from build123d import *

# Parameters (mm, degrees)
SKETCH1_W                                  = 38
SKETCH1_H                                  = 18
BOSS_EXTRUDE1_DEPTH                        = 34
BOSS_EXTRUDE2_START                        = -6
SKETCH2_W                                  = 54
SKETCH2_H                                  = 18
BOSS_EXTRUDE2_DEPTH                        = 2
CUT_EXTRUDE1_DEPTH                         = 48
CUT_EXTRUDE1_DEPTH_BACK                    = 48
SKETCH3_W                                  = 1.5
SKETCH3_H                                  = 1
SKETCH4_R                                  = 6
BOSS_EXTRUDE3_DEPTH                        = 1.5
SKETCH5_W                                  = 6
SKETCH5_H                                  = 2
BOSS_EXTRUDE4_DEPTH                        = 1
FILLET1_RADIUS                             = 1
FILLET1_LENGTH                             = 1
FILLET1_OF_MIRROR1_2_RADIUS                = 1
FILLET1_OF_MIRROR1_2_LENGTH                = 1
SKETCH6_W                                  = 7
SKETCH6_H                                  = 4
BOSS_EXTRUDE5_DEPTH                        = 5
SKETCH7_R                                  = 3
BOSS_EXTRUDE6_DEPTH                        = 4
BOSS_EXTRUDE7_START                        = 8
SKETCH8_R                                  = 7
BOSS_EXTRUDE7_DEPTH                        = 2
SKETCH9_R                                  = 4
BOSS_EXTRUDE8_DEPTH                        = 4
SKETCH10_R                                 = 2.25
CUT_EXTRUDE2_DEPTH                         = 4
MIRROR2_AT_THE_SECOND_PLANE_COPY_1_SKETC_R = 2.25
MIRROR2_AT_THE_SECOND_PLANE_COPY_1_DEPTH   = 4


with BuildPart() as part:
    # Sketch1 → Boss-Extrude1 (new body)
    with BuildSketch(Plane(origin=(0, 0, 0), x_dir=(1, 0, 0), z_dir=(0, 1, 0))):
        Rectangle(SKETCH1_W, SKETCH1_H)
    extrude(amount=BOSS_EXTRUDE1_DEPTH)

    # Sketch2 → Boss-Extrude2 (add)
    with BuildSketch(Plane(origin=(0, 34, 0), x_dir=(1, 0, 0), z_dir=(0, 1, 0)).offset(BOSS_EXTRUDE2_START)):
        Rectangle(SKETCH2_W, SKETCH2_H)
    extrude(amount=-BOSS_EXTRUDE2_DEPTH)

    # Sketch3 → Cut-Extrude1 (cut, two sides: drawn at the far end of the back side and taken through both)
    with BuildSketch(Plane.XY.offset(9).offset(-CUT_EXTRUDE1_DEPTH_BACK)):
        Polygon((-19, 30), (-16, 31), (-14, 34), (-19, 34), align=None)
        with Locations((-1.75, 33.5)):
            Rectangle(SKETCH3_W, SKETCH3_H)
    extrude(amount=CUT_EXTRUDE1_DEPTH + CUT_EXTRUDE1_DEPTH_BACK, mode=Mode.SUBTRACT)

    # Sketch4 → Boss-Extrude3 (add)
    with BuildSketch(Plane(origin=(0, 34, 0), x_dir=(1, 0, 0), z_dir=(0, 1, 0))):
        with Locations(Location((10, 0, 0), (0, 0, 90))):
            Circle(SKETCH4_R)
    extrude(amount=BOSS_EXTRUDE3_DEPTH)

    # Sketch5 → Boss-Extrude4 (add)
    with BuildSketch(Plane(origin=(0, 28, 0), x_dir=(1, 0, 0), z_dir=(0, 1, 0))):
        with Locations((-22, 0)):
            Rectangle(SKETCH5_W, SKETCH5_H)
    boss_extrude4 = extrude(amount=BOSS_EXTRUDE4_DEPTH)

    # Fillet1: full round fillet: the end face becomes a half cylinder, R = half its width
    fillet1_face = Plane((-25, 28.5, 0), x_dir=(0, -1, 0), z_dir=(-1, 0, 0))  # on the end face: x along it, z out of the body
    fillet1_slab = fillet1_face.offset(-FILLET1_RADIUS / 2) * Box(FILLET1_LENGTH, 2 * FILLET1_RADIUS, FILLET1_RADIUS, mode=Mode.PRIVATE)  # the body's end, R deep
    fillet1_round = Plane((-24, 28.5, 0), x_dir=(-1, 0, 0), z_dir=(0, -1, 0)) * Cylinder(FILLET1_RADIUS, FILLET1_LENGTH, mode=Mode.PRIVATE)  # its axis R under the face
    add(fillet1_slab - fillet1_round, mode=Mode.SUBTRACT)

    # Mirror1: Boss-Extrude4 across plane
    add(boss_extrude4.mirror(Plane(origin=(0, 0, 0), x_dir=(0, 0, 1), z_dir=(1, 0, 0))))

    # Fillet1 of Mirror1 2: full round fillet: the end face becomes a half cylinder, R = half its width
    fillet1_of_mirror1_2_face = Plane((25, 28.5, 0), x_dir=(0, -1, 0), z_dir=(1, 0, 0))  # on the end face: x along it, z out of the body
    fillet1_of_mirror1_2_slab = fillet1_of_mirror1_2_face.offset(-FILLET1_OF_MIRROR1_2_RADIUS / 2) * Box(FILLET1_OF_MIRROR1_2_LENGTH, 2 * FILLET1_OF_MIRROR1_2_RADIUS, FILLET1_OF_MIRROR1_2_RADIUS, mode=Mode.PRIVATE)  # the body's end, R deep
    fillet1_of_mirror1_2_round = Plane((24, 28.5, 0), x_dir=(1, 0, 0), z_dir=(0, -1, 0)) * Cylinder(FILLET1_OF_MIRROR1_2_RADIUS, FILLET1_OF_MIRROR1_2_LENGTH, mode=Mode.PRIVATE)  # its axis R under the face
    add(fillet1_of_mirror1_2_slab - fillet1_of_mirror1_2_round, mode=Mode.SUBTRACT)

    # Sketch6 → Boss-Extrude5 (add)
    with BuildSketch(Plane(origin=(19, 0, 0), x_dir=(0, 0, -1), z_dir=(1, 0, 0))):
        with Locations((0, 3)):
            Rectangle(SKETCH6_W, SKETCH6_H)
    extrude(amount=BOSS_EXTRUDE5_DEPTH)

    # Sketch7 → Boss-Extrude6 (add)
    with BuildSketch(Plane(origin=(0, 35.5, 0), x_dir=(1, 0, 0), z_dir=(0, 1, 0))):
        with Locations(Location((10, 0, 0), (0, 0, 270))):
            Circle(SKETCH7_R)
    extrude(amount=BOSS_EXTRUDE6_DEPTH)



with BuildPart() as body_2:
    # Sketch8 → Boss-Extrude7 (new body)
    with BuildSketch(Plane(origin=(0, 34, 0), x_dir=(1, 0, 0), z_dir=(0, 1, 0)).offset(BOSS_EXTRUDE7_START)):
        with Locations(Location((10, 0, 0), (0, 0, 270))):
            Circle(SKETCH8_R)
    extrude(amount=-BOSS_EXTRUDE7_DEPTH)


with BuildPart() as part_1:
    add(part.part)

    add(body_2.part)  # Boss-Extrude8 merges body 2
    # Sketch9 → Boss-Extrude8 (add)
    with BuildSketch(Plane.XZ.offset(-40)):
        with Locations(Location((10, 0, 0), (0, 0, 270))):
            Circle(SKETCH9_R)
    extrude(amount=BOSS_EXTRUDE8_DEPTH)

    # Sketch10 → Cut-Extrude2 (cut)
    with BuildSketch(Plane(origin=(0, 28, 0), x_dir=(1, 0, 0), z_dir=(0, 1, 0))):
        with Locations(Location((-23.25, 5, 0), (0, 0, 270))):
            Circle(SKETCH10_R)
    cut_extrude2 = extrude(amount=-CUT_EXTRUDE2_DEPTH, mode=Mode.SUBTRACT)

    # Mirror2: Cut-Extrude2 across plane
    add(cut_extrude2.mirror(Plane.XY), mode=Mode.SUBTRACT)

    # Mirror2 at the second plane: Cut-Extrude2 across plane
    add(cut_extrude2.mirror(Plane(origin=(0, 0, 0), x_dir=(0, 0, 1), z_dir=(1, 0, 0))), mode=Mode.SUBTRACT)

    # Mirror2 at the second plane copy 1 sketc → Mirror2 at the second plane copy 1 (cut)
    with BuildSketch(Plane(origin=(0, 28, 0), x_dir=(-1, 0, 0), z_dir=(0, 1, 0))):
        with Locations(Location((-23.25, 5, 0), (0, 0, 270))):
            Circle(MIRROR2_AT_THE_SECOND_PLANE_COPY_1_SKETC_R)
    extrude(amount=-MIRROR2_AT_THE_SECOND_PLANE_COPY_1_DEPTH, mode=Mode.SUBTRACT)


solid = part_1.part
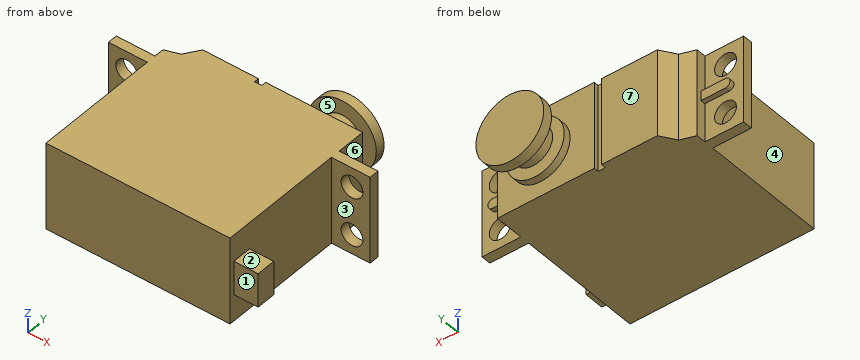
CAD build for the part. Positions are in the model's coordinates, mm. Face numbers are marked on the shaded views. A direction names the side the tool comes from. Coordinates: 2 decimals unless noted, no trailing zeros. Write each loop counter-clockwise with the first axis right and the second up, starting at its lowest first coordinate (ties: lowest second). Pieces come first, ordered by that corner, then holes. Notation, with made-up numbers: M -23,27.5 L -18,27.5 A19 cw -18,47.5 Z; hole C -21,20.5 d2. An arc over 180 degrees is marked long. Answer as a JSON object with one key per item and string values. Group by question number.
1) Tool access for the marked faces 1, 2, 3 and 4: list every direction of +Z, -Z, +X, -X, +Y, -Y with a clear straight run to the whole face (end or side of a thin tool).
2) Saw through at A-A (x = -23.25). Write the cut outline in (y, z).
3) Wall check: line 1 (X direction, y = 26.55, z = 5); line 2 (Z direction, x = -23, y = 27); line 3 (Y direction, x = 8, z = 3.5). Give the ranges that are in metal, low to high. Write a range as from..to.
4) Saw through at C-C (z = 5). Give the number of separate pieces and of enclosed holes in the cut face, plus the area to 3 significant figures.
5) Mould opens along Y. For the marked faces 5, 6 and 7 say: +Y half, -Y half, draft (parallel to the pull), parting line (faces both ways), or undercut.
6) Saw through at B-B (x = 23.25). Write the cut outline in (y, z), plus the area to 3 significant figures.
7) Pin check, flat tips, straight feed: pin 1 Ø1.5 at (y, z) = (12, 7) entering from +X; pin 2 Ø6 at (x, z) = (23.25, -5) entering from +Y; pin 3 Ø1.5 at (x, z) = (22, 0) entering from -Y; pin 4 Ø8 at (y, z) = (30.5, -4.5) entering from -X. Stop position of each tip, or through.
8) Saw through at D-D (y = 12). Write the cut outline in (x, z).
Values follow:
{
 "1": {"face 1": "+Z, -Z, +X, -Y", "face 2": "+Z, +X, -Y", "face 3": "+Z, -Z, +X", "face 4": "+Z, -Z, -X, -Y"},
 "2": {"outline": "M 26,-9 L 28,-9 L 28,-7.25 L 26,-7.25 Z; M 26,-2.75 L 28,-2.75 L 28,-1 L 29,-1 L 29,1 L 28,1 L 28,2.75 L 26,2.75 Z; M 26,7.25 L 28,7.25 L 28,9 L 26,9 Z"},
 "3": {"line 1": "x = -27..-25.5, -21..21, 25.5..27", "line 2": "z = -9..-7.24, -2.76..2.76, 7.24..9", "line 3": "y = 0..35.5, 40..42"},
 "4": {"separate pieces": "4", "enclosed holes": "0", "area": "1,320 mm2"},
 "5": {"face 5": "undercut", "face 6": "draft", "face 7": "+Y half"},
 "6": {"outline": "M 1,-3.5 L 5,-3.5 L 5,3.5 L 1,3.5 Z; M 26,-9 L 28,-9 L 28,-7.25 L 26,-7.25 Z; M 26,-2.75 L 28,-2.75 L 28,-1 L 29,-1 L 29,1 L 28,1 L 28,2.75 L 26,2.75 Z; M 26,7.25 L 28,7.25 L 28,9 L 26,9 Z", "area": "48.0 mm2"},
 "7": {"pin 1": "stops at x = 19", "pin 2": "stops at y = 28", "pin 3": "stops at y = 1", "pin 4": "stops at x = -27"},
 "8": {"outline": "M -19,-9 L 19,-9 L 19,9 L -19,9 Z"}
}
